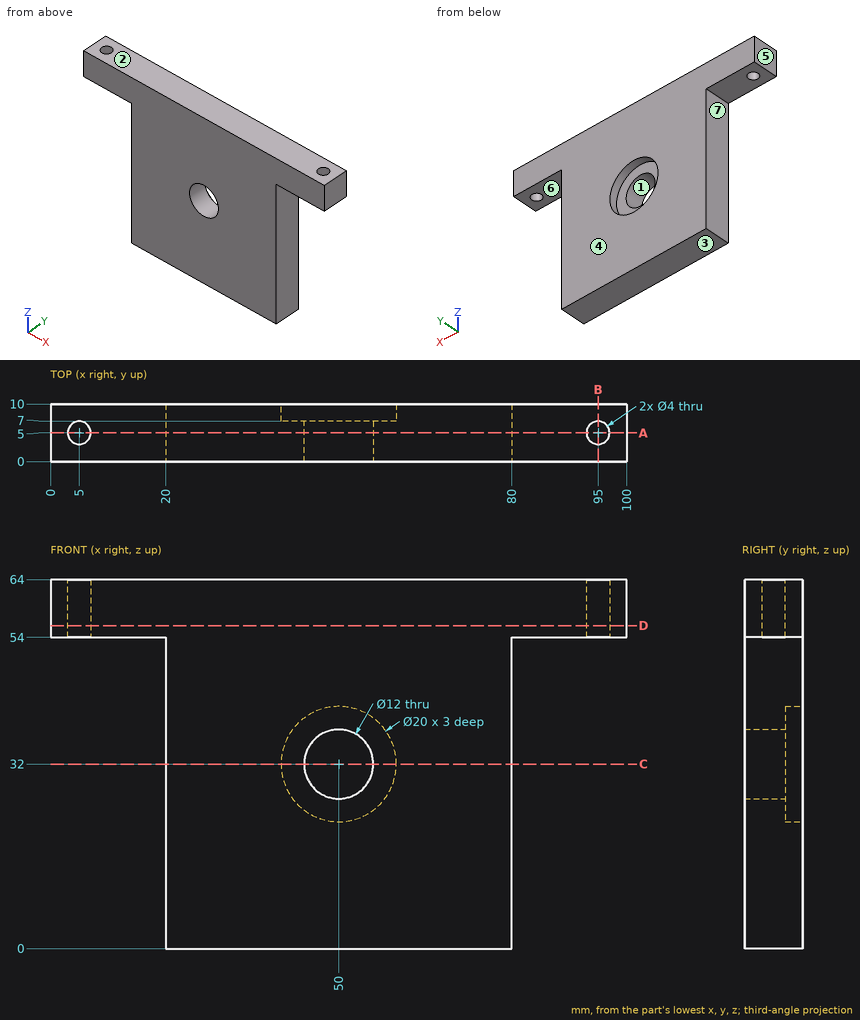
Check sheet for the drawn part. Datum: minimum x, y, z corner. Units: mm. A direction names the side the tool comes from. Round coordinates to 2 decimals unless told otherwise and drop trailing zeros. Loops run counter-clockwise (first coordinate to the right, second up) from the corner with the lowest first, then second, coordinate; pieces in that order, holes last. Notation, with made-up numbers: (-40, -2) - (19, -2) arc R19 ccw to (19, 17) - close; hole circle Ø6 at (-36, -28). An arc over 180 degrees is marked (long way). Answer as a JSON object with one key per item and string values. Group by question number.
Q1. Sectioned sample at B-B, the plane x = 95. Enter the section's corners in (y, z), plus the area to 3 significant figures.
Q2. Sectioned sample at C-C, the plane z = 32. Enter the section's corners in (x, y).
Q3. Set-up check for the marked faces 5, 6 and 7: record each of +Z, -Z, +X, -X, +Y, -Y from which the full face is reachable in a straight line by a thin tool's end or side.
Q4. Mould release check, pull along Z, two halves, no side actions. Record for the marked faces 1, 2, 3 and 4: released by +Z, released by -Z, zero draft, split by the parting line, or undercut.
Q5. Gauge pin test, flat ends, axial feed: P1, Ø19, axis at x = 50, z = 32, coming from the +Y side; P2, Ø23, axis at x = 50, z = 32, coming from the +Y side; P3, Ø5, axis at x = 92, y = 3, coming from the -Z side; P4, Ø1.5, axis at y = 1, z = 45, coming from the -X side. Record the tip position at first contact, or that the pin passes through.
Q6. Sectioned sample at D-D, the plane z = 56. Enter the section's corners in (x, y), plus the area to 3 significant figures.
Q7. Scan lines: line 1 along Z through (x, y) = (50, 7.8); line 2 along Y through (x, z) = (5, 58); line 3 along X through (y, z) = (3.75, 55). Record each from-to range of solid material in increasing order. Write a range as [from, to].
Q8. Sectioned sample at A-A, the plane y = 5. Enter the section's corners in (x, z), plus the area to 3 significant figures.
Solution:
{
 "1": {"outline": "(0, 54) - (3, 54) - (3, 64) - (0, 64) - close; (7, 54) - (10, 54) - (10, 64) - (7, 64) - close", "area": "60.0 mm²"},
 "2": {"outline": "(20, 0) - (44, 0) - (44, 7) - (40, 7) - (40, 10) - (20, 10) - close; (56, 0) - (80, 0) - (80, 10) - (60, 10) - (60, 7) - (56, 7) - close"},
 "3": {"face 5": "+Z, -Z, -X, +Y, -Y", "face 6": "-Z, +X, +Y, -Y", "face 7": "-Z, -X, +Y, -Y"},
 "4": {"face 1": "undercut", "face 2": "released by +Z", "face 3": "released by -Z", "face 4": "zero draft"},
 "5": {"P1": "stops at y = 7", "P2": "stops at y = 10", "P3": "stops at z = 54", "P4": "stops at x = 20"},
 "6": {"outline": "(0, 0) - (100, 0) - (100, 10) - (0, 10) - close; hole circle Ø4 at (5, 5); hole circle Ø4 at (95, 5)", "area": "975 mm²"},
 "7": {"line 1": "z = [0, 22], [42, 64]", "line 2": "y = [0, 3], [7, 10]", "line 3": "x = [0, 3.44], [6.56, 93.44], [96.56, 100]"},
 "8": {"outline": "(0, 54) - (3, 54) - (3, 64) - (0, 64) - close; (7, 54) - (20, 54) - (20, 0) - (80, 0) - (80, 54) - (93, 54) - (93, 64) - (7, 64) - close; (97, 54) - (100, 54) - (100, 64) - (97, 64) - close; hole circle Ø12 at (50, 32)", "area": "4,050 mm²"}
}
